from build123d import *

# Parameters (mm, degrees)
SKETCH1_R                = 75
SKETCH1_R_2              = 40
BOSS_EXTRUDE1_DEPTH      = 60
BOSS_EXTRUDE2_START      = 30
SKETCH2_R                = 40
SKETCH2_R_2              = 10
BOSS_EXTRUDE2_DEPTH      = 15
BOSS_EXTRUDE2_DEPTH_BACK = 15
SKETCH5_R                = 25
SKETCH5_R_2              = 2
SKETCH5_R_3              = 4
BOSS_EXTRUDE4_DEPTH      = 5
BOSS_EXTRUDE5_START      = -30
SKETCH5_2_R              = 25
SKETCH5_2_R_2            = 2
SKETCH5_2_R_3            = 4
BOSS_EXTRUDE5_DEPTH      = 5
SKETCH6_R                = 10
SKETCH6_R_2              = 4
BOSS_EXTRUDE6_DEPTH      = 15
BOSS_EXTRUDE7_START      = -40
SKETCH6_2_R              = 10
SKETCH6_2_R_2            = 4
BOSS_EXTRUDE7_DEPTH      = 15


with BuildPart() as part:
    # Sketch1 → Boss-Extrude1 (new body)
    with BuildSketch(Plane.XY):
        Circle(SKETCH1_R)
        Circle(SKETCH1_R_2, mode=Mode.SUBTRACT)
    extrude(amount=BOSS_EXTRUDE1_DEPTH)

    # Sketch2 → Boss-Extrude2 (add, two sides)
    with BuildSketch(Plane.XY.offset(BOSS_EXTRUDE2_START)) as boss_extrude2_sk:
        Circle(SKETCH2_R)
        Circle(SKETCH2_R_2, mode=Mode.SUBTRACT)
        Polygon((7.5, 35), (-7.5, 35), (-3, 15), (3, 15), align=None, mode=Mode.SUBTRACT)
        Polygon((30.969350613, 17.948518675), (13.338796761, 7.488424465), (15.192898728, 1.782085367), (35.604605528, 3.682670931), align=None, mode=Mode.SUBTRACT)
        Polygon((26.640111288, -23.907205411), (11.243829768, -10.371899159), (6.389727801, -13.898610672), (14.504856372, -32.723984195), align=None, mode=Mode.SUBTRACT)
        Polygon((-14.504856372, -32.723984195), (-6.389727801, -13.898610673), (-11.243829768, -10.371899159), (-26.640111288, -23.907205411), align=None, mode=Mode.SUBTRACT)
        Polygon((-35.604605528, 3.682670931), (-15.192898728, 1.782085367), (-13.338796761, 7.488424465), (-30.969350613, 17.948518675), align=None, mode=Mode.SUBTRACT)
    extrude(amount=BOSS_EXTRUDE2_DEPTH)
    extrude(boss_extrude2_sk.sketch, amount=-BOSS_EXTRUDE2_DEPTH_BACK)

    # Sketch5 → Boss-Extrude4 (add)
    with BuildSketch(Plane.XY.offset(45)):
        with Locations(Location((0, 0, 0), (0, 0, 173.841878739))):
            Circle(SKETCH5_R)
        with Locations((-11.040892983, 14.216141605)):
            Circle(SKETCH5_R_2, mode=Mode.SUBTRACT)
        with Locations((10.108530546, 14.893542567)):
            Circle(SKETCH5_R_2, mode=Mode.SUBTRACT)
        with Locations((17.288308436, -5.011426086)):
            Circle(SKETCH5_R_2, mode=Mode.SUBTRACT)
        with Locations((0.576231676, -17.990774221)):
            Circle(SKETCH5_R_2, mode=Mode.SUBTRACT)
        with Locations((-16.932177675, -6.107483866)):
            Circle(SKETCH5_R_2, mode=Mode.SUBTRACT)
        Circle(SKETCH5_R_3, mode=Mode.SUBTRACT)
    extrude(amount=BOSS_EXTRUDE4_DEPTH)

    # Sketch5_2 → Boss-Extrude5 (add)
    with BuildSketch(Plane.XY.offset(45).offset(BOSS_EXTRUDE5_START)):
        with Locations(Location((0, 0, 0), (0, 0, 173.841878739))):
            Circle(SKETCH5_2_R)
        with Locations((-11.040892983, 14.216141605)):
            Circle(SKETCH5_2_R_2, mode=Mode.SUBTRACT)
        with Locations((10.108530546, 14.893542567)):
            Circle(SKETCH5_2_R_2, mode=Mode.SUBTRACT)
        with Locations((17.288308436, -5.011426086)):
            Circle(SKETCH5_2_R_2, mode=Mode.SUBTRACT)
        with Locations((0.576231676, -17.990774221)):
            Circle(SKETCH5_2_R_2, mode=Mode.SUBTRACT)
        with Locations((-16.932177675, -6.107483866)):
            Circle(SKETCH5_2_R_2, mode=Mode.SUBTRACT)
        Circle(SKETCH5_2_R_3, mode=Mode.SUBTRACT)
    extrude(amount=-BOSS_EXTRUDE5_DEPTH)

    # Sketch6 → Boss-Extrude6 (add)
    with BuildSketch(Plane(origin=(0, 0, 10), x_dir=(-1, 0, 0), z_dir=(0, 0, -1))):
        with Locations(Location((0, 0, 0), (0, 0, 180))):
            Circle(SKETCH6_R)
        with Locations(Location((0, 0, 0), (0, 0, 180))):
            Circle(SKETCH6_R_2, mode=Mode.SUBTRACT)
    extrude(amount=BOSS_EXTRUDE6_DEPTH)

    # Sketch6_2 → Boss-Extrude7 (add)
    with BuildSketch(Plane(origin=(0, 0, 10), x_dir=(-1, 0, 0), z_dir=(0, 0, -1)).offset(BOSS_EXTRUDE7_START)):
        with Locations(Location((0, 0, 0), (0, 0, 180))):
            Circle(SKETCH6_2_R)
        Circle(SKETCH6_2_R_2, mode=Mode.SUBTRACT)
    extrude(amount=-BOSS_EXTRUDE7_DEPTH)


solid = part.part
Work out the finished part from the listing and answer in its coordinate system (mm). A direction names the side the tool comes from. Give positions to 0.01 mm unless a question says otherwise; leave off trailing zeros. Order: outer loops, then holes, each group sorted by start corner. A loop starts at its lowest first (then second) coordinate and runs counter-clockwise, first axis right, second up. Notation, with made-up numbers: (63.25, 31) -> (90.25, 31) arc R31 ccw to (90.25, 61) -> close; hole circle Ø10 at (31.25, 52.5). An arc over 180 degrees is marked (long way). Answer as a JSON object with one key per item and string values. Group by question number.
1. Section A-A on z = 32 is taken. Determine the outline of the cut face in (x, y), plus the area to 3 significant figures.
2. Flat-ended cylindrical pins translate along their axes: pin 1 Ø5 at (y, z) = (-58.5, 3) entering from -X; pin 2 Ø4.5 at (x, y) = (-16.93, -6.11) entering from +Z; pin 3 Ø12 at (y, z) = (44, 2.5) entering from -X; pin 4 Ø12 at (x, y) = (0, 0) entering from +Z. Find the tip coordinate at first contact, or state that the pin passes through.
3. Consider line 1 along Y through (x, z) = (0, 33.75); line 2 along Y through (x, z) = (0, 56); line 3 along X through (y, z) = (-0.5, 27). Determine where each line is inside the solid, lowest interval first. Write a range as [from, to].
4. Section C-C on x = -42.5 is taken. Determine the outline of the cut face in (y, z).
5. A tool of negligible diameter and unlimited length cuts with its end or side. For faces 4 (the flat face through (-25.542, 2.746, 29.79)), 5 (the flat face through (-20.66, -28.25, 30.21)), 6 (the cylindrical face through (12.016, 15.494, 12.535)), 7 (the flat face through (-17, -6, 45)), from which of +Z, -Z, +X, -X, +Y, -Y can it reach the whole face along a straight path? Write none if from no direction.
6. The mould has two halves that part along Z. Classify faces 1 (the flat face through (17.22, 18.34, 45)), 2 (the flat face through (0, 20, 45)), 3 (the flat face through (2, 11, 10)): released by +Z, released by -Z, zero draft, split by the parting line, or undercut.
7. Section B-B on y = -60 is taken. Determine the outline of the cut face in (x, z).
Result sheet:
{
 "1": {"outline": "circle Ø150 at (0, 0); hole (-35.6, 3.68) -> (-15.19, 1.78) -> (-13.34, 7.49) -> (-30.97, 17.95) -> close; hole (-26.64, -23.91) -> (-14.5, -32.72) -> (-6.39, -13.9) -> (-11.24, -10.37) -> close; hole circle Ø20 at (0, 0); hole (-7.5, 35) -> (-3, 15) -> (3, 15) -> (7.5, 35) -> close; hole (6.39, -13.9) -> (14.5, -32.72) -> (26.64, -23.91) -> (11.24, -10.37) -> close; hole (13.34, 7.49) -> (15.19, 1.78) -> (35.6, 3.68) -> (30.97, 17.95) -> close", "area": "16,300 mm^2"},
 "2": {"pin 1": "stops at x = -49.89", "pin 2": "stops at z = 50", "pin 3": "stops at x = -64.66", "pin 4": "stops at z = 65"},
 "3": {"line 1": "y = [-75, -10], [10, 15], [35, 75]", "line 2": "y = [-75, -40], [-10, -4], [4, 10], [40, 75]", "line 3": "x = [-75, -9.99], [9.99, 75]"},
 "4": {"outline": "(-61.8, 0) -> (61.8, 0) -> (61.8, 60) -> (-61.8, 60) -> close"},
 "5": {"face 4": "none", "face 5": "+Z, -Z", "face 6": "-Z", "face 7": "+Z"},
 "6": {"face 1": "released by +Z", "face 2": "undercut", "face 3": "released by -Z"},
 "7": {"outline": "(-45, 0) -> (45, 0) -> (45, 60) -> (-45, 60) -> close"}
}
